```python
from build123d import *

# Parameters (mm, degrees)
F0_R     = 2
F0_R_2   = 3
F1_DEPTH = 5
F2_R     = 0.2
F3_SIZE  = 1


with BuildPart() as f1:
    # F0 (on Front) → F1 (new body)
    with BuildSketch(Plane.XZ):
        Polygon((-21.416343, -9.780747), (-21.416343, -21.780747), (20.583657, -21.780747), (20.583657, -9.780747), (7.621113, 21.219253), (-7.929415, 21.219253), align=None)
        with Locations((-17, -15.780747)):
            Circle(F0_R, mode=Mode.SUBTRACT)
        with Locations((17, -15.780747)):
            Circle(F0_R, mode=Mode.SUBTRACT)
        with Locations((0, 15.219253)):
            Circle(F0_R_2, mode=Mode.SUBTRACT)
    extrude(amount=F1_DEPTH)

    # F2
    f2_edges = [f1.edges().sort_by_distance(p)[0] for p in [
        (-14.672879, -5, 5.719253),
        (-0.154151, -5, 21.219253),
        (14.102385, -5, 5.719253),
        (14.102385, 0, 5.719253),
        (-0.154151, 0, 21.219253),
        (7.621113, -2.5, 21.219253),
        (-7.929415, -2.5, 21.219253),
        (-14.672879, 0, 5.719253),
    ]]
    fillet(f2_edges, radius=F2_R)

    # F3
    f3_edges = [f1.edges().sort_by_distance(p)[0] for p in [
        (-19, -5, -15.780747),
        (15, -5, -15.780747),
    ]]
    chamfer(f3_edges, length=F3_SIZE)


solid = f1.part
```
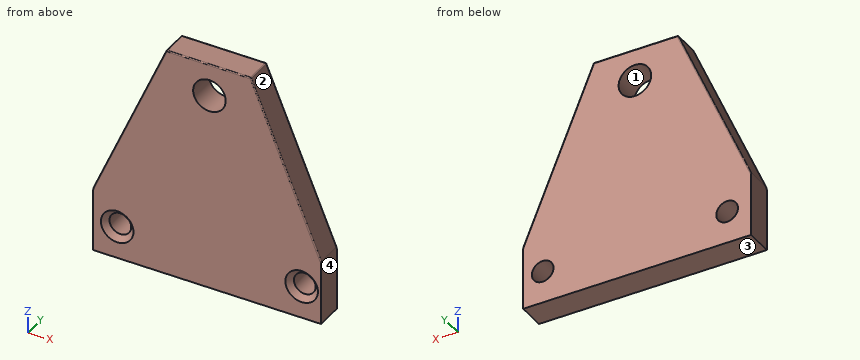
Geometry check sheet. Reference: the model listing, model coordinates, mm. Face numbers are marked on the shaded views. Coordinates: 2 decimals unless noted, no trailing zeros. Order: outer loops, then holes, each group sorted by start corner. A loop starts at its lowest first (then second) coordinate and runs counter-clockwise, first axis right, second up. Notation, with made-up numbers: (4, -27.5) - (43, -27.5) arc R21 ccw to (43, 3.5) - close; hole circle Ø5 at (-24.5, 58). An arc over 180 degrees is marked (long way). Answer in a Markdown table with one row per item. Add a question column.
1. Section check A-A (x = 0). Enter the section's corners in (y, z), plus the area to 3 significant figures.
2. Draft check along Z on the marked faces 1, 2, 3 and 4. Enter one of: +Z half, -Z half, draft (parallel to the pull), parting line (faces both ways), or undercut.
3. Material ranges on L1, parallel to X at y = -1.2, z = -14; L2, parallel to X at y = -2.9, z = -15; L3, parallel to Z at x = 18, y = -4.55 (3 decimals), recorded low to high. Write a range as [from, to].
4. Gauge pin test, flat ends, axial feed: pin 1 Ø2.5 at (x, z) = (17, -15.78) entering from -Y; pin 2 Ø5 at (x, z) = (-17, -15.78) entering from -Y. Record the tip position at first contact, or that the pin passes through.
5. Section check B-B (y = -1.4). Enter the section's corners in (x, z).
Data:
| question | item | result |
|---|---|---|
| 1 | outline | (-5, -21.78) - (0, -21.78) - (0, 12.22) - (-5, 12.22) - close; (-5, 18.22) - (0, 18.22) - (0, 21.02) arc R0.2 ccw to (-0.2, 21.22) - (-4.8, 21.22) arc R0.2 ccw to (-5, 21.02) - close |
| 1 | area | 185 mm² |
| 2 | face 1 | undercut |
| 2 | face 2 | +Z half |
| 2 | face 3 | -Z half |
| 2 | face 4 | draft |
| 3 | L1 | x = [-21.42, -17.91], [-16.09, 16.09], [17.91, 20.58] |
| 3 | L2 | x = [-21.42, -18.84], [-15.16, 15.16], [18.84, 20.58] |
| 3 | L3 | z = [-21.781, -18.126], [-13.435, -3.602] |
| 4 | pin 1 | passes through |
| 4 | pin 2 | stops at y = -4.5 |
| 5 | outline | (-21.42, -21.78) - (20.58, -21.78) - (20.58, -9.78) - (7.67, 21.1) arc R0.2 ccw to (7.49, 21.22) - (-7.8, 21.22) arc R0.2 ccw to (-7.98, 21.1) - (-21.42, -9.78) - close; hole circle Ø4 at (-17, -15.78); hole circle Ø6 at (0, 15.22); hole circle Ø4 at (17, -15.78) |
